from build123d import *

# Parameters (mm, degrees)
BOSS_EXTRUDE1_DEPTH = 300
SKETCH2_R           = 23.25
CUT_EXTRUDE1_DEPTH  = 10
SKETCH3_R           = 7
CUT_EXTRUDE2_DEPTH  = 10


with BuildPart() as part:
    # Sketch1 → Boss-Extrude1 (new body)
    with BuildSketch(Plane.XY):
        Polygon((0, -37.5), (0, 37.5), (75, 37.5), (75, 31.15), (6.35, 31.15), (6.35, -31.15), (75, -31.15), (75, -37.5), align=None)
    extrude(amount=BOSS_EXTRUDE1_DEPTH)

    # Sketch2 → Cut-Extrude1 (cut)
    with BuildSketch(Plane(origin=(0, 37.5, 0), x_dir=(1, 0, 0), z_dir=(0, 1, 0))):
        with Locations(Location((40, -150, 0), (0, 0, 270))):
            Circle(SKETCH2_R)
    extrude(amount=-CUT_EXTRUDE1_DEPTH, mode=Mode.SUBTRACT)

    # Sketch3 → Cut-Extrude2 (cut)
    with BuildSketch(Plane.XZ.offset(37.5)):
        with Locations(Location((40, 150, 0), (0, 0, 270))):
            Circle(SKETCH3_R)
    extrude(amount=-CUT_EXTRUDE2_DEPTH, mode=Mode.SUBTRACT)


solid = part.part
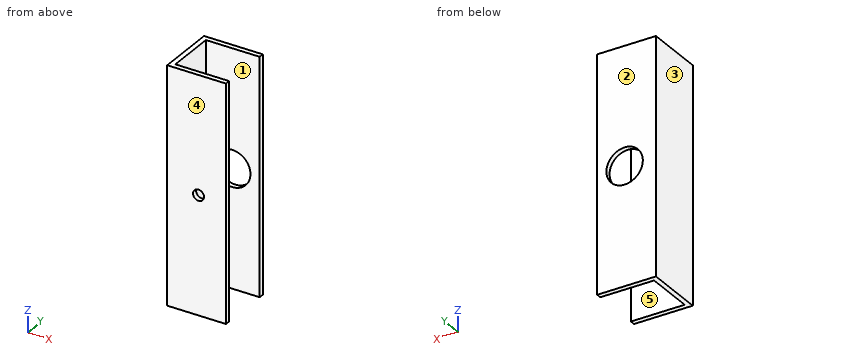
Geometry check sheet. Reference: the model listing, model coordinates, mm. Face numbers are marked on the shaded views. A direction names the side the tool comes from. Give positions to 0.01 mm unless a question says otherwise; leave off trailing zeros. Write each loop counter-clockwise with the first axis right and the second up, starting at its lowest first coordinate (ties: lowest second). Pieces come first, ordered by that corner, then holes. Notation, with made-up numbers: M 39.5,89.5 L 54.5,89.5 A27 ccw 54.5,120.5 Z; hole C -24,-1 d10. An arc over 180 degrees is marked long. One line per question, with ' | ' between items.
1. Cross-section at B-B (z = 150). Enter the section's corners in (x, y), plus the area to 3 significant figures.
Ans:
outline: M 0,-37.5 L 33,-37.5 L 33,-31.15 L 6.35,-31.15 L 6.35,31.15 L 16.75,31.15 L 16.75,37.5 L 0,37.5 Z; M 47,-37.5 L 75,-37.5 L 75,-31.15 L 47,-31.15 Z; M 63.25,31.15 L 75,31.15 L 75,37.5 L 63.25,37.5 Z | area: 964 mm2
2. Scan lines: line 1 along X through (y, z) = (36, 150); line 2 along Y through (x, z) = (17.5, 247); line 3 along X through (y, z) = (-35, 150). Record each from-to range of solid material in increasing order. Write a range as from..to.
Ans:
line 1: 0..16.75, 63.25..75 | line 2: -37.5..-31.15, 31.15..37.5 | line 3: 0..33, 47..75
3. Cross-section at C-C (x = 24.5). Enter the section's corners in (y, z), plus the area to 3 significant figures.
Ans:
outline: M -37.5,0 L -31.15,0 L -31.15,300 L -37.5,300 Z; M 31.15,0 L 37.5,0 L 37.5,132.67 L 31.15,132.67 Z; M 31.15,167.33 L 37.5,167.33 L 37.5,300 L 31.15,300 Z | area: 3,590 mm2
4. Cross-section at D-D (y = 9). Enter the section's corners in (x, z).
Ans:
outline: M 0,0 L 6.35,0 L 6.35,300 L 0,300 Z
5. Set-up check for the marked faces 1 and 2: record each of +Z, -Z, +X, -X, +Y, -Y from which the full face is reachable in a straight line by a thin tool's end or side.
Ans:
face 1: +Z, -Z, +X | face 2: +Z, -Z, +X, -X, +Y
6. Cross-section at A-A (x = 40). Enter the section's corners in (y, z), plus the area to 3 significant figures.
Ans:
outline: M -37.5,0 L -31.15,0 L -31.15,143 L -37.5,143 Z; M -37.5,157 L -31.15,157 L -31.15,300 L -37.5,300 Z; M 31.15,0 L 37.5,0 L 37.5,126.75 L 31.15,126.75 Z; M 31.15,173.25 L 37.5,173.25 L 37.5,300 L 31.15,300 Z | area: 3,430 mm2
7. Gauge pin test, flat ends, axial feed: pin 1 (8 mm diameter, centred on x = 62.5, y = -28.5, fed in from +Z); pin 2 (6 mm diameter, centred on y = -20, z = 156, fed in from +X). Record the tip position at first contact, or that the pin passes through.
Ans:
pin 1: z = 300 | pin 2: x = 6.35
8. Mould release check, pull along Y, two halves, no side actions. Record for the marked faces 3, 4 and 5: released by +Y, released by -Y, zero draft, split by the parting line, or undercut.
Ans:
face 3: zero draft | face 4: released by -Y | face 5: undercut
